Input: part model. Units: mm. Frame: model coordinates. A direction names the side the tool comes from. Round coordinates to 2 decimals unless told otherwise and drop trailing zeros. Loops run counter-clockwise (first coordinate to the right, second up) from the corner with the lowest first, then second, coordinate; pieces in that order, holes last. Notation, with made-up numbers: (34, 17.25) -> (56, 17.25) arc R23 ccw to (56, 55.25) -> close; hole circle Ø9 at (78, -1). An arc over 180 degrees is marked (long way). Answer in a Markdown table with one row per item. Add a question column.
Q1. Section D-D, the plane y = 172. Output: boundary loops of the cut face in (x, z), and give its area (3 significant figures).
Q2. Reachability of faces 1 (the face through (7.5, 8, 8)), 2 (the face through (0, 49, 85)), 3 (the face through (-129.5, 161, -100)) from +Z, -Z, +X, -X, +Y, -Y: full face, straight path, thin tool, end or side. Return the list, or none.
Q3. Section B-B, the plane z = -92. Output: boundary loops of the cut face in (x, y).
Q4. Mould query, pull axis Y, two halves, no side actions, for faces 4 (the face through (-39, 150, 105)), 5 (the face through (0, 49, -85)), 6 (the face through (-145, 110, 100)), 7 (the face through (0, 10, 1)). Classes: pulls with the +Y half, pulls with the -Y half, needs draft (parallel to the pull), parting line crosses it, or undercut.
Q5. Section C-C, the plane x = -21. Output: boundary loops of the cut face in (y, z).
Q6. Section A-A, the plane y = 47.5. Output: boundary loops of the cut face in (x, z), and give its area (3 significant figures).
Q7. Pin query (flat end, axial travel): pin 1 (3 mm diameter, centred on x = -141.25, y = 186.75, fed in from +Z); pin 2 (9 mm diameter, centred on x = -151.5, y = 159, fed in from +Z); pin 3 (1.5 mm diameter, centred on x = -102, z = -56, fed in from -Y); pin 4 (3 mm diameter, centred on x = -93.5, z = 61.5, fed in from +Y). Return the tip coordinate at first contact, or that it passes through.
Q8. Ray query, L1, parallel to Y at x = -141.25, z = 91; L2, parallel to Z at x = 3, y = 6; L3, parallel to Z at x = 15.5, y = 156. Return the intervals inside material, ascending. Write a range as from..to.
Autodesk Inventor part; units mm, degrees
ref_plane "YZ Plane" through (0, 0, 0) normal (1, 0, 0) x (0, 1, 0)
ref_plane "XZ Plane" through (0, 0, 0) normal (0, 1, 0) x (-1, 0, 0)
ref_plane "XY Plane" through (0, 0, 0) normal (0, 0, 1) x (1, 0, 0)
sketch "Boceto2" plane through (0, 0, 0) normal (0, 1, 0) x (-1, 0, 0)
  line L0 (7.5, 105) -> (-7.5, 105)
  line L1 (-7.5, 105) -> (-7.5, -105)
  line L2 (-7.5, -105) -> (7.5, -105)
  line L3 (7.5, -105) -> (7.5, 105)
  line L4 (7.5, 105) -> (-7.5, -105) construction
  line L5 (-7.5, 105) -> (7.5, -105) construction
  point P0 (0, 0)
  dimension "d7" = 15
  dimension "d8" = 210
extrude "Extrusión1" add sketch "Boceto2" along normal blind 10
sketch "Boceto3" plane through (0, 10, 0) normal (0, 1, 0) x (1, 0, 0)
  line L0 (5, 60) -> (-5, 60)
  line L1 (-5, 60) -> (-5, 70)
  line L2 (-5, 70) -> (5, 70)
  line L3 (5, 70) -> (5, 60)
  line L4 (5, 60) -> (-5, 70) construction
  line L5 (7.5, 105) -> (-7.5, 105)
  line L6 (0, 64.5148) -> (0, 61.9205)
  circle A0 centre (3.25, 61.75) radius 1.75
  circle A1 centre (-3.25, 68.25) radius 1.75
  line L7 (-7.5, 105) -> (-7.5, -105)
  line L8 (-7.5, 0) -> (0, 0)
  line L9 (5, -70) -> (5, -60)
  line L10 (-5, -70) -> (5, -70)
  line L11 (5, -60) -> (-5, -60)
  line L12 (-5, -60) -> (-5, -70)
  line L13 (5, -60) -> (-5, -70) construction
  line L14 (0, -64.5148) -> (0, -61.9205)
  circle A2 centre (-3.25, -68.25) radius 1.75
  circle A3 centre (3.25, -61.75) radius 1.75
  point P0 (3.25, 68.25)
  point P1 (-5, 65)
  point P2 (-3.25, 61.75)
  point P3 (0, 105)
  point P4 (3.25, -68.25)
  point P5 (-3.25, -61.75)
  point P6 (-5, -65)
  dimension "d12" = 1.75
  dimension "d13" = 1.75
  dimension "d14" = 1.75
  dimension "d15" = 1.75
  dimension "d16" = 10
  dimension "d17" = 10
  dimension "d19" = 35
  dimension "d67" = 36.75
hole "Agujero1" at (3.25, 10, -61.75) at (-3.25, 10, -68.25) at (-3.25, 10, 68.25) at (3.25, 10, 61.75) direction (0, -1, 0) diameter 3.5 end through all
sketch "Boceto4" plane through (0, 10, 0) normal (0, 1, 0) x (1, 0, 0)
  line L0 (-7.5, 105) -> (-7.5, -105)
  line L1 (-7.5, -105) -> (7.5, -105)
  line L2 (7.5, -105) -> (7.5, -85)
  line L3 (7.5, -85) -> (-7.5, -85)
  line L4 (-7.5, -85) -> (-7.5, -105)
  line L5 (-7.5, 0) -> (1.0116, 0)
  line L6 (-7.5, -105) -> (-7.5, 105)
  line L7 (-7.5, 105) -> (7.5, 105)
  line L8 (7.5, 105) -> (7.5, 85)
  line L9 (7.5, 85) -> (-7.5, 85)
  line L10 (-7.5, 85) -> (-7.5, 105)
  point P0 (0, 0)
  dimension "d27" = 15
  dimension "d28" = 20
extrude "Extrusión2" add sketch "Boceto4" along normal blind 80
sketch "Boceto5" plane through (0, 90, 0) normal (0, 1, 0) x (1, 0, 0)
  line L0 (-7.5, -105) -> (7.5, -105)
  line L1 (-7.5, -105) -> (40.5, -105)
  line L2 (40.5, -105) -> (40.5, 105)
  line L3 (40.5, 105) -> (-7.5, 105)
  line L4 (-7.5, 105) -> (-7.5, -105)
  line L5 (40.5, -105) -> (-159.5, -105)
  line L6 (-159.5, -105) -> (-159.5, 105)
  line L7 (-159.5, 105) -> (40.5, 105)
  line L8 (40.5, 105) -> (40.5, -105)
  point P0 (0, 0)
  dimension "d31" = 48
  dimension "d32" = 200
extrude "Extrusión3" add sketch "Boceto5" along normal blind 120
sketch "Boceto6" plane through (0, 210, 0) normal (0, 1, 0) x (1, 0, 0)
  line L0 (40.5, 105) -> (7.5, 105)
  line L1 (40.5, 105) -> (20.5, 105)
  line L2 (20.5, 105) -> (20.5, 85)
  line L3 (7.5, -105) -> (40.5, -105)
  line L4 (24, -105) -> (24, -85)
  line L5 (-159.5, 105) -> (-159.5, -105)
  line L6 (20.5, 85) -> (-159.5, 85)
  line L7 (-159.5, 85) -> (-159.5, -85)
  line L8 (-159.5, -85) -> (20.5, -85)
  line L9 (20.5, -85) -> (20.5, 85)
  point P0 (7.5, 85)
  dimension "d36" = 20
  dimension "d37" = 20
  dimension "d38" = 20
extrude "Extrusión4" cut sketch "Boceto6" against normal blind 100
sketch "Boceto7" plane through (-159.5, 90, -105) normal (-1, 0, 0) x (0, 0, 1)
  line L0 (0, 120) -> (20, 120)
  line L1 (20, 120) -> (10, 120)
  line L2 (10, 120) -> (10, 20)
  line L3 (10, 20) -> (20, 20)
  line L4 (20, 20) -> (20, 120)
  line L5 (190, 120) -> (190, 20)
  line L6 (190, 120) -> (200, 120)
  line L7 (200, 120) -> (200, 20)
  line L8 (200, 20) -> (190, 20)
  line L9 (190, 20) -> (190, 120)
  line L10 (210, 0) -> (210, 120)
  line L11 (0, 0) -> (0, 120)
  line L12 (0, 120) -> (10, 120)
  line L13 (10, 120) -> (10, 20)
  line L14 (10, 20) -> (0, 20)
  line L15 (0, 20) -> (0, 120)
  line L16 (210, 120) -> (0, 120)
  line L17 (210, 120) -> (200, 120)
  line L18 (200, 120) -> (200, 20)
  line L19 (200, 20) -> (210, 20)
  line L20 (210, 20) -> (210, 120)
  point P0 (105, -90)
  dimension "d42" = 10
  dimension "d63" = 10
  dimension "d65" = 10
extrude "Extrusión5" cut sketch "Boceto7" against normal blind 30 contours L0 L2 L14 L11 | L16 L10 L19 L7
sketch "Boceto8" plane through (-7.5, 0, 105) normal (0, 0, 1) x (1, 0, 0)
  line L0 (-122, 210) -> (-122, 110)
  line L1 (-132, 185) -> (-142, 185)
  line L2 (-142, 185) -> (-142, 195)
  line L3 (-142, 195) -> (-132, 195)
  line L4 (-132, 195) -> (-132, 185)
  line L5 (-132, 185) -> (-142, 195) construction
  line L6 (-142, 185) -> (-132, 195) construction
  line L7 (-152, 210) -> (48, 210)
  line L8 (-113, 160) -> (-128, 160)
  line L9 (-152, 110) -> (-122, 110)
  line L10 (-132, 190) -> (-131.5898, 190)
  circle A0 centre (-140.25, 193.25) radius 1.75
  circle A1 centre (-133.75, 186.75) radius 1.75
  line L11 (-132, 125) -> (-132, 135)
  line L12 (-142, 125) -> (-132, 125)
  line L13 (-132, 135) -> (-142, 125) construction
  line L14 (-132, 135) -> (-142, 135)
  line L15 (-142, 135) -> (-132, 125) construction
  line L16 (-142, 135) -> (-142, 125)
  line L17 (-132, 130) -> (-131.5898, 130)
  circle A2 centre (-133.75, 133.25) radius 1.75
  circle A3 centre (-140.25, 126.75) radius 1.75
  line L18 (-152, 110) -> (-152, 210)
  point P0 (7.5, 0)
  point P1 (-113, 215)
  point P2 (-133.75, 193.25)
  point P3 (-142, 190)
  point P4 (-140.25, 186.75)
  point P5 (48, 210)
  point P6 (-133.75, 126.75)
  point P7 (-140.25, 133.25)
  point P8 (-143, 115)
  point P9 (-133.75, 126.75)
  point P10 (-140.25, 133.25)
  point P11 (-142, 130)
  dimension "d46" = 1.75
  dimension "d47" = 1.75
  dimension "d48" = 1.75
  dimension "d49" = 1.75
  dimension "d50" = 10
  dimension "d51" = 10
  dimension "d52" = 15
  dimension "d66" = 10
  dimension "d70" = 15
hole "Agujero2" at (-147.75, 193.25, 105) at (-141.25, 186.75, 105) at (-147.75, 126.75, 105) at (-141.25, 133.25, 105) direction (0, 0, -1) diameter 3.5 end through all
properties part number "container_back"
Answer block:
| question | item | result |
|---|---|---|
| 1 | outline | (-159.5, -95) -> (-129.5, -95) -> (-129.5, -105) -> (40.5, -105) -> (40.5, 105) -> (-129.5, 105) -> (-129.5, 95) -> (-159.5, 95) -> (-159.5, 85) -> (20.5, 85) -> (20.5, -85) -> (-159.5, -85) -> close |
| 1 | area | 10,800 mm^2 |
| 2 | face 1 | +Z, -Z, +X, -Y |
| 2 | face 2 | +X, -X |
| 2 | face 3 | -Z, -X, +Y |
| 3 | outline | (-159.5, 90) -> (-7.5, 90) -> (-7.5, 0) -> (7.5, 0) -> (7.5, 90) -> (40.5, 90) -> (40.5, 210) -> (-159.5, 210) -> close; hole circle Ø3.5 at (-147.75, 126.75); hole circle Ø3.5 at (-147.75, 193.25); hole circle Ø3.5 at (-141.25, 133.25); hole circle Ø3.5 at (-141.25, 186.75) |
| 4 | face 4 | needs draft |
| 4 | face 5 | undercut |
| 4 | face 6 | pulls with the +Y half |
| 4 | face 7 | undercut |
| 5 | outline | (90, -105) -> (210, -105) -> (210, -85) -> (110, -85) -> (110, 85) -> (210, 85) -> (210, 105) -> (90, 105) -> close |
| 6 | outline | (-7.5, -105) -> (7.5, -105) -> (7.5, -85) -> (-7.5, -85) -> close; (-7.5, 85) -> (7.5, 85) -> (7.5, 105) -> (-7.5, 105) -> close |
| 6 | area | 600 mm^2 |
| 7 | pin 1 | through |
| 7 | pin 2 | z = 95 |
| 7 | pin 3 | y = 90 |
| 7 | pin 4 | y = 110 |
| 8 | L1 | 90..131.5, 135..185, 188.5..210 |
| 8 | L2 | -105..-63.48, -60.02..60.02, 63.48..105 |
| 8 | L3 | -105..-85, 85..105 |
